from build123d import *

# Parameters (mm, degrees)
REVOLUCI_N2_ANGLE     = 270
CROQUIS12_R           = 10.307991632
CORTAR_EXTRUIR1_DEPTH = 67.177507085
CROQUIS12_2_R         = 10.307991632
CORTAR_EXTRUIR2_DEPTH = 97.177507085


with BuildPart() as part:
    # Croquis2 → Revolución2 (revolve)
    with BuildSketch(Plane.XY):
        with BuildLine():
            Line((-25, 0), (-25, 15))
            Line((-25, 15), (75, 15))
            Line((75, 15), (75, 30))
            Line((75, 30), (55, 30))
            Line((55, 30), (55, 51.3))
            Line((55, 51.3), (45, 51.3))
            Line((45, 51.3), (45, 36.3))
            Line((45, 36.3), (40, 36.3))
            Line((40, 36.3), (40, 56.246772292))
            ThreePointArc((40, 56.246772292), (38.76797888, 57.241607231), (37.5, 58.19018625))
            Line((37.5, 58.19018625), (37.5, 36.3))
            Line((37.5, 36.3), (32.5, 36.3))
            Line((32.5, 36.3), (32.5, 61.290245221))
            ThreePointArc((32.5, 61.290245221), (31.259906067, 61.920128903), (30, 62.509385314))
            Line((30, 62.509385314), (30, 36.3))
            Line((30, 36.3), (25, 36.3))
            Line((25, 36.3), (25, 64.384554711))
            ThreePointArc((25, 64.384554711), (23.755157932, 64.744183719), (22.5, 65.065965261))
            Line((22.5, 65.065965261), (22.5, 36.3))
            Line((22.5, 36.3), (17.5, 36.3))
            Line((17.5, 36.3), (17.5, 65.957524099))
            ThreePointArc((17.5, 65.957524099), (16.251612737, 66.085843567), (15, 66.177507085))
            Line((15, 66.177507085), (15, 36.3))
            Line((15, 36.3), (10, 36.3))
            Line((10, 36.3), (10, 66.177507085))
            ThreePointArc((10, 66.177507085), (8.748387263, 66.085843567), (7.5, 65.957524099))
            Line((7.5, 65.957524099), (7.5, 36.3))
            Line((7.5, 36.3), (2.5, 36.3))
            Line((2.5, 36.3), (2.5, 65.065965261))
            ThreePointArc((2.5, 65.065965261), (1.244842068, 64.744183719), (0, 64.384554711))
            Line((0, 64.384554711), (0, 36.3))
            Line((0, 36.3), (-5, 36.3))
            Line((-5, 36.3), (-5, 62.509385314))
            ThreePointArc((-5, 62.509385314), (-6.259906067, 61.920128903), (-7.5, 61.290245221))
            Line((-7.5, 61.290245221), (-7.5, 36.3))
            Line((-7.5, 36.3), (-12.5, 36.3))
            Line((-12.5, 36.3), (-12.5, 58.19018625))
            ThreePointArc((-12.5, 58.19018625), (-13.76797888, 57.241607231), (-15, 56.246772292))
            Line((-15, 56.246772292), (-15, 36.3))
            Line((-15, 36.3), (-20, 36.3))
            Line((-20, 36.3), (-20, 51.3))
            Line((-20, 51.3), (-35, 51.3))
            Line((-35, 51.3), (-49.922676306, 41.234527738))
            Line((-49.922676306, 41.234527738), (-49.922676306, 20))
            ThreePointArc((-49.922676306, 20), (-52.851608494, 12.928932188), (-59.922676306, 10))
            Line((-59.922676306, 10), (-65, 10))
            Line((-65, 10), (-65, 20))
            Line((-65, 20), (-75, 20))
            Line((-75, 20), (-75, 0))
            Line((-75, 0), (-25, 0))
        make_face()
    revolve(axis=Axis((-75, -15, 0), (1, 0, 0)), revolution_arc=REVOLUCI_N2_ANGLE)

    # Croquis12 → Cortar-Extruir1 (cut, through all)
    with BuildSketch(Plane(origin=(0, 0, 0), x_dir=(1, 0, 0), z_dir=(0, 1, 0))):
        with Locations((35, 0)):
            Circle(CROQUIS12_R)
    extrude(amount=CORTAR_EXTRUIR1_DEPTH, mode=Mode.SUBTRACT)

    # Croquis12<2> → Cortar-Extruir2 (cut, through all)
    with BuildSketch(Plane(origin=(0, 0, 0), x_dir=(1, 0, 0), z_dir=(0, 1, 0))):
        with Locations((35, 0)):
            Circle(CROQUIS12_2_R)
    extrude(amount=-CORTAR_EXTRUIR2_DEPTH, mode=Mode.SUBTRACT)


solid = part.part
CAD build for the part. Positions are in the model's coordinates, mm. A direction names the side the tool comes from. Give positions to 0.01 mm unless a question says otherwise; leave off trailing zeros. Write each loop counter-clockwise with the first axis right and the second up, starting at its lowest first coordinate (ties: lowest second). Pieces come first, ordered by that corner, then holes. Notation, with made-up numbers: (0.25, 0.5) -> (12.25, 0.5) arc R26 ccw to (12.25, 38.5) -> close; hole circle Ø9 at (77, -18.75). An arc over 180 degrees is marked (long way). Return JSON: item names as keys, results as strings.
Item 1: Tool access for faces 4 (the flat face through (-25, -21, 14)), 5 (the cylindrical face through (-27.6, -60.31, 48.4)), 6 (the cylindrical face through (27.46, -13.91, 51.29)), 7 (the flat face through (10, -68, 19)), 8 (the flat face through (-1, -15, -41)): list every direction of +Z, -Z, +X, -X, +Y, -Y with a clear straight run to the whole face (end or side of a thin tool).
Answer below:
{"face 4": "+X", "face 5": "-X", "face 6": "+Z", "face 7": "none", "face 8": "-Z, +X, -X, +Y"}
Item 2: Two-plate mould, pull along Y, no slides. Class faces 1 (the flat face through (-65, -33, 18)), 2 (the cylindrical face through (4.96, -50.06, 37.45)), 3 (the cylindrical face through (25.7, -35.502, 21.901)): +Y half, -Y half, draft (parallel to the pull), parting line (faces both ways), or undercut.
Answer below:
{"face 1": "draft", "face 2": "parting line", "face 3": "undercut"}
Item 3: Drop flat-ended pins along their axis: pin 1 (1.5 mm diameter, centred on x = 3, z = -65, fed in from +Y); pin 2 (2 mm diameter, centred on x = 50.5, z = 22, fed in from -Y); pin 3 (1 mm diameter, centred on x = 8.5, z = -3.5, fed in from +Y). Give the stop position or say it passes through.
Answer below:
{"pin 1": "stops at y = -15", "pin 2": "stops at y = -77.89", "pin 3": "stops at y = -44.73"}
Item 4: Drill centre lines: probe 1 along X at (y, z) = (-58.5, 0); probe 2 along Z at (x, y) = (35, -54.5); probe 3 along X at (y, z) = (20, 9). Where is each one in solid material? Low to high.
Answer below:
{"probe 1": "x = -49.92 to 24.69, 45.31 to 75", "probe 2": "z = -32.73 to -10.31, 10.31 to 32.73", "probe 3": "x = -49.92 to 29.97, 40.03 to 75"}
Item 5: Band-saw the part on C-C (x = -40.5). List the corners of the cut face in (y, z).
Answer below:
{"outline": "(-15, -62.59) -> (-15, -15) arc R15 cw (long way) to (0, 0) -> (47.59, 0) arc R62.59 ccw (long way) to start"}
Item 6: Band-saw the part on B-B (x = -22.5). List the corners of the cut face in (y, z).
Answer below:
{"outline": "(-15, -66.3) -> (-15, -30) arc R30 cw (long way) to (15, 0) -> (51.3, 0) arc R66.3 ccw (long way) to start"}
Item 7: Band-saw the part on A-A (x = 35). List the corners of the cut face in (y, z), then the cut area to 3 significant figures.
Answer below:
{"outline": "(-65.25, -10.31) arc R51.3 ccw to (-15, -51.3) -> (-15, -30) arc R30 cw to (-43.17, -10.31) -> close; (-65.25, 10.31) -> (-43.17, 10.31) arc R30 cw to (13.17, 10.31) -> (35.25, 10.31) arc R51.3 ccw to start", "area": "3,410 mm2"}
